The figure shows three views and two pictorial views of one solid part (mm, origin at its lowest corner). Answer the questions. Give positions to 0.01 mm unless a question says otherwise; leave off trailing zeros. Write each loop counter-clockwise with the first axis right and the second up, starting at its lowest first coordinate (ties: lowest second). Pieces come first, ordered by that corner, then holes. Notation, with made-up numbers: (62.25, 77.25) - (113.25, 77.25) arc R27 ccw to (113.25, 102.25) - close; hole circle Ø10 at (-25, 28). An arc over 180 degrees is marked (long way). Use a Markdown table: item, result. Add a question column.
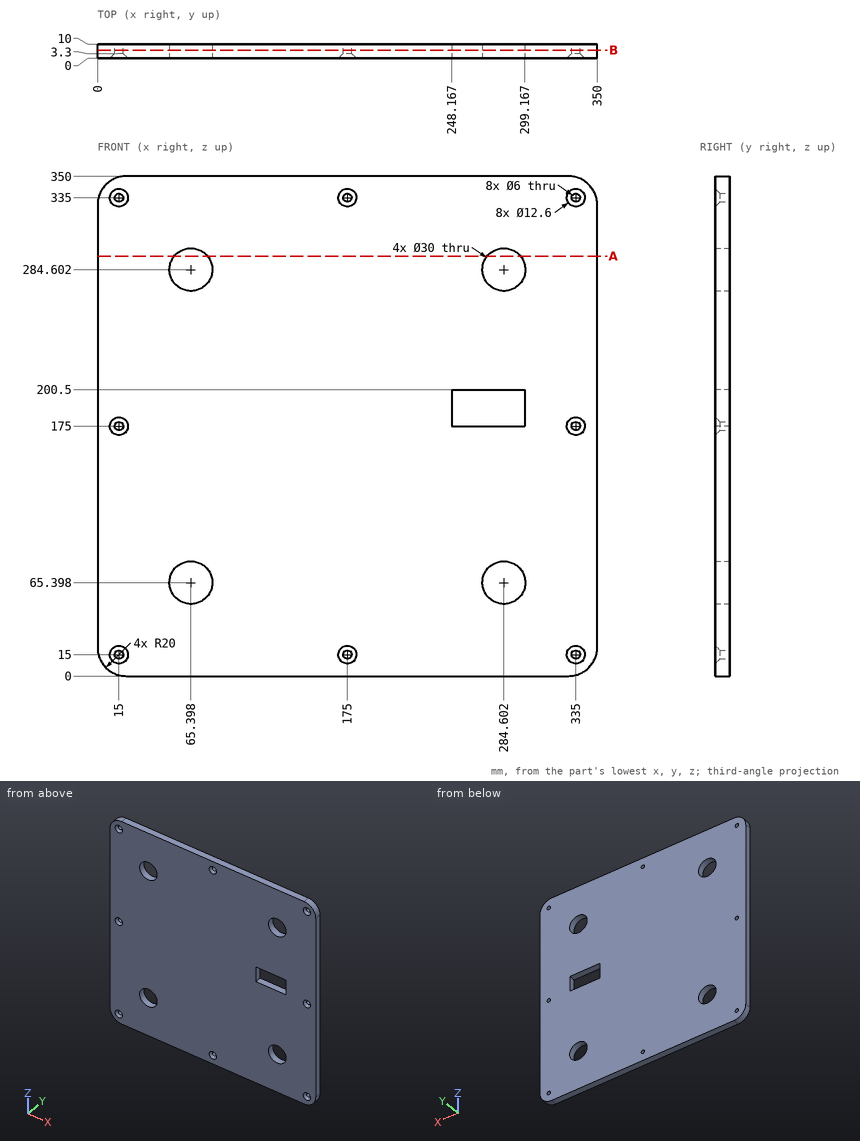
1. Consider L1, parallel to X at y = 6.5, z = 191.5; L2, parallel to Z at x = 175, y = 7.75; L3, parallel to Z at x = 335, y = 5 (1 decimal). Determine where each line is inside the solid, lowest interval first. Write a range as [from, to].
2. Given P1, Ø5, axis at x = 335, z = 335, coming from the -Y side; P2, Ø7, axis at x = 335, z = 15, coming from the -Y side; P3, Ø8, axis at x = 15, z = 175, coming from the -Y side, each flat-ended and moving along its own axis, determine where each tip first touches the part or whether it passes through.
3. The part is cut by section B-B (y = 5.75). Count the separate pieces of the cut face and the enclosed holes in it, and give its area (3 significant figures).
4. The part is cut by section A-A (z = 294). Give the vertices of the cut face in (x, y), and give its area (3 significant figures).
Check values:
| question | item | result |
|---|---|---|
| 1 | L1 | x = [0, 248.17], [299.17, 350] |
| 1 | L2 | z = [0, 12], [18, 332], [338, 350] |
| 1 | L3 | z = [0.6, 12], [18, 172], [178, 332], [338, 349.4] |
| 2 | P1 | passes through |
| 2 | P2 | stops at y = 2.8 |
| 2 | P3 | stops at y = 2.3 |
| 3 | separate pieces | 1 |
| 3 | enclosed holes | 13 |
| 3 | area | 118,000 mm2 |
| 4 | outline | (0, 0) - (53.71, 0) - (53.71, 10) - (0, 10) - close; (77.09, 0) - (272.91, 0) - (272.91, 10) - (77.09, 10) - close; (296.29, 0) - (350, 0) - (350, 10) - (296.29, 10) - close |
| 4 | area | 3,030 mm2 |
